The listing builds one solid part. Answer for the finished solid, in the listing's coordinates (mm). Give positions to 0.01 mm unless a question says otherwise; leave off trailing zeros. Write each loop counter-clockwise with the first axis right and the second up, starting at its lowest first coordinate (ties: lowest second). Pieces come first, ordered by that corner, then holes. Notation, with made-up numbers: (65.25, 37) - (117.25, 37) arc R20 ccw to (117.25, 76) - close; hole circle Ø3 at (-17.5, 67.5). An arc over 180 degrees is marked (long way). One line per question, with ' | ' between items. Start each with the question number.
1. Given P1, Ø4, axis at x = 84, y = -109.5, coming from the -Z side; P2, Ø1.5, axis at x = 49, z = 24.5, coming from the -Y side; P3, Ø1.5, axis at x = 86, z = 22.5, coming from the -Y side, each flat-ended and moving along its own axis, determine where each tip first touches the part or whether it passes through.
2. A cutting plane is placed at C-C (y = -50). Determine the outline of the cut face in (x, z), then the cut area to 3 significant figures.
3. Find the intervals of material crossed by L1, parallel to Y at x = 12, z = 59; L2, parallel to X at y = -53.5, z = 52; L3, parallel to X at y = -68, z = 60, in increasing order. Write a range as from..to.
4. The mould has two halves that part along Y. Classify faces 1 (the face through (43.726, -145.684, 30.864)), 2 (the face through (47.637, -79.466, 32.883)), 3 (the face through (50, 0, 33)): +Y half, -Y half, draft (parallel to the pull), parting line (faces both ways), or undercut.
5. A cutting plane is placed at B-B (z = 47). Determine the outline of the cut face in (x, y).
6. A cutting plane is placed at D-D (y = -74). Determine the outline of the cut face in (x, z).
7. A cutting plane is placed at A-A (x = 65). Determine the outline of the cut face in (y, z), then the cut area to 3 significant figures.
```python
from build123d import *

# Parameters (mm, degrees)
F0_W         = 102.258592844
F0_H         = 64.8588836193
F1_DEPTH     = 111.87066
F2_R         = 22.1566524367
F3_DEPTH     = 123.47648
F4_R         = 18.3530030386
F5_DEPTH     = 205.67378
F6_T1_DEPTH  = 140.358592844
F6_T3_DEPTH  = 102.9588836193
F6_T5_DEPTH  = 149.97066
F6_S9_W      = 25.4
F6_S9_H      = 25.4
F6_T10_DEPTH = 25.4
F7_R         = 10.8823528673
F8_DEPTH     = 68.58648


# Not quite as in the source:
# - a fillet or chamfer that OpenCascade refuses, or shapes differently, is made with other operations: its cross-section is extruded or revolved along the edge and cut away or added


with BuildPart() as f1:
    # F0 (on Front) → F1 (new body)
    with BuildSketch(Plane.XZ):
        with Locations((51.129296422, 32.4294418097)):
            Rectangle(F0_W, F0_H)
    extrude(amount=F1_DEPTH)

    # F2 (on face) → F3 (cut)
    with BuildSketch(Plane.XY.offset(64.8588836193)):
        with Locations((52.4399839342, -57.8363165259)):
            Circle(F2_R)
    extrude(amount=-F3_DEPTH, mode=Mode.SUBTRACT)

    # F4 (on face) → F5 (cut)
    with BuildSketch(Plane.YZ.offset(102.258592844)):
        with Locations((-52.9614761472, 32.6913073659)):
            Circle(F4_R)
    extrude(amount=-F5_DEPTH, mode=Mode.SUBTRACT)

    # F6: fillet of radius 25.4 on 3 edges, made by hand

    # F6_s2 → F6_t1 (cut)
    with BuildSketch(Plane.YZ.offset(-63.5)):
        with BuildLine():
            ThreePointArc((-111.87066, 25.4), (-104.4311722421, 7.4394877579), (-86.47066, 0))
            Line((-86.47066, 0), (-111.87066, 0))
            Line((-111.87066, 0), (-111.87066, 25.4))
        make_face()
    extrude(amount=F6_T1_DEPTH, mode=Mode.SUBTRACT)

    # F6_s4 → F6_t3 (cut)
    with BuildSketch(Plane.XY.offset(25.4)):
        with BuildLine():
            ThreePointArc((76.858592844, -111.87066), (94.8191050861, -104.4311722421), (102.258592844, -86.47066))
            Line((102.258592844, -86.47066), (102.258592844, -111.87066))
            Line((102.258592844, -111.87066), (76.858592844, -111.87066))
        make_face()
    extrude(amount=F6_T3_DEPTH, mode=Mode.SUBTRACT)

    # F6_s6 → F6_t5 (cut)
    with BuildSketch(Plane.XZ.offset(-63.5)):
        with BuildLine():
            ThreePointArc((76.858592844, 0), (94.8191050861, 7.4394877579), (102.258592844, 25.4))
            Line((102.258592844, 25.4), (102.258592844, 0))
            Line((102.258592844, 0), (76.858592844, 0))
        make_face()
    extrude(amount=F6_T5_DEPTH, mode=Mode.SUBTRACT)


with BuildPart() as f6_tool8:
    # F6_s9 → F6_t10 (new body)
    with BuildSketch(Plane.XZ.offset(86.47066)):
        with Locations((89.558592844, 12.7)):
            Rectangle(F6_S9_W, F6_S9_H)
    extrude(amount=F6_T10_DEPTH)

    # F6_s11 → F6_t12 (revolve, cut)
    with BuildSketch(Plane(origin=(76.858592844, -86.47066, 25.4), x_dir=(-0.7071067812, 0, 0.7071067812), z_dir=(0.7071067812, 0, 0.7071067812))):
        with BuildLine():
            ThreePointArc((0, -25.4), (25.4, 0), (0, 25.4))
            Line((0, 25.4), (0, -25.4))
        make_face()
    revolve(axis=Axis((76.858592844, -86.47066, 25.4), (0, -1, 0)), mode=Mode.SUBTRACT)


with BuildPart() as f1_1:
    add(f1.part)

    # F6_t7: cut F6_tool8
    add(f6_tool8.part, mode=Mode.SUBTRACT)

    # F7 (on face) → F8 (join)
    with BuildSketch(Plane.XZ.offset(111.87066)):
        with Locations((38.7039594352, 40.518656373)):
            Circle(F7_R)
    extrude(amount=F8_DEPTH)


solid = f1_1.part
```
Determined:
1) P1: z = 12.9 | P2: y = -111.87 | P3: y = -110.28
2) outline: (0, 0) - (31.72, 0) - (31.72, 14.58) - (0, 14.58) - close; (0, 50.8) - (31.72, 50.8) - (31.72, 64.86) - (0, 64.86) - close; (73.16, 0) - (76.86, 0) arc R25.4 ccw to (99.84, 14.58) - (73.16, 14.58) - close; (73.16, 50.8) - (102.26, 50.8) - (102.26, 64.86) - (73.16, 64.86) - close | area: 1,610 mm2
3) L1: -111.87..0 | L2: 0..30.71, 74.17..102.26 | L3: 0..32.75, 72.13..102.26
4) face 1: draft | face 2: undercut | face 3: +Y half
5) outline: (0, -111.87) - (29.96, -111.87) - (29.96, -180.46) - (47.45, -180.46) - (47.45, -111.87) - (76.86, -111.87) arc R25.4 ccw to (102.26, -86.47) - (102.26, -64.45) - (73.59, -64.45) arc R22.16 cw to (31.29, -64.45) - (0, -64.45) - close; (0, -41.47) - (37.51, -41.47) arc R22.16 cw to (67.37, -41.47) - (102.26, -41.47) - (102.26, 0) - (0, 0) - close
6) outline: (0, 0) - (37.29, 0) - (37.29, 64.86) - (0, 64.86) - close; (67.59, 0) - (76.86, 0) arc R25.4 ccw to (102.26, 25.4) - (102.26, 64.86) - (67.59, 64.86) - close
7) outline: (-111.87, 25.4) arc R25.4 ccw to (-86.47, 0) - (-76.09, 0) - (-76.09, 64.86) - (-111.87, 64.86) - close; (-39.58, 0) - (0, 0) - (0, 64.86) - (-39.58, 64.86) - (-39.58, 45.26) arc R18.35 cw to (-39.58, 20.13) - close | area: 4,660 mm2
